Read the model definition and answer for the solid it produces. Units are mm, in the model's axes. Face numbers are marked on the shaded views. A direction names the side the tool comes from. Round coordinates to 2 decimals unless told otherwise and drop trailing zeros. Loops run counter-clockwise (first coordinate to the right, second up) from the corner with the lowest first, then second, coordinate; pieces in that order, holes last. Notation, with made-up numbers: M 46.25,-12.5 L 82.25,-12.5 A12 cw 82.25,-6.5 Z; hole C 38.25,-10.5 d7. An arc over 180 degrees is marked long. Write each question's results on one line, items separated by ' | '.
from build123d import *

# Parameters (mm, degrees)
SKETCH2_W           = 57
SKETCH2_H           = 120.75
SKETCH2_W_2         = 51
SKETCH2_H_2         = 114.75
BOSS_EXTRUDE1_DEPTH = 75
SKETCH3_W           = 57
SKETCH3_H           = 120.75
BOSS_EXTRUDE2_DEPTH = 3
SKETCH4_W           = 78
SKETCH4_H           = 57
BOSS_EXTRUDE3_DEPTH = 5
SKETCH6_R           = 2.675
CUT_EXTRUDE2_DEPTH  = 10
CUT_EXTRUDE3_DEPTH  = 138.287528874
BOSS_EXTRUDE4_REACH = 139.288
CUT_EXTRUDE7_DEPTH  = 150.745739841
BOSS_EXTRUDE8_DEPTH = 5
SKETCH21_R          = 3
CUT_EXTRUDE11_DEPTH = 1094
CHAMFER2_SIZE       = 2
CHAMFER2_SIZE2      = 6.751886845
SKETCH22_R          = 1.675
CUT_EXTRUDE12_DEPTH = 1094
CUT_EXTRUDE13_DEPTH = 5
SKETCH25_R          = 5.125
CUT_EXTRUDE14_DEPTH = 131.551099899
CHAMFER3_SIZE       = 2
FILLET1_R           = 2
SKETCH27_R          = 3
CUT_EXTRUDE15_DEPTH = 3
CUT_EXTRUDE16_DEPTH = 10


with BuildPart() as part:
    # Sketch2 → Boss-Extrude1 (new body)
    with BuildSketch(Plane(origin=(0, 0, 0), x_dir=(0, 0, -1), z_dir=(1, 0, 0))):
        with Locations((2.896243414, -39.494242434)):
            Rectangle(SKETCH2_W, SKETCH2_H)
        with Locations((2.896243414, -39.494242434)):
            Rectangle(SKETCH2_W_2, SKETCH2_H_2, mode=Mode.SUBTRACT)
    extrude(amount=BOSS_EXTRUDE1_DEPTH)

    # Sketch3 → Boss-Extrude2 (add)
    with BuildSketch(Plane.ZY):
        with Locations((-2.896243414, -39.494242434)):
            Rectangle(SKETCH3_W, SKETCH3_H)
    extrude(amount=BOSS_EXTRUDE2_DEPTH)

    # Sketch4 → Boss-Extrude3 (add)
    with BuildSketch(Plane(origin=(0, 20.880757566, 0), x_dir=(1, 0, 0), z_dir=(0, 1, 0))):
        with Locations((36, 2.896243414)):
            Rectangle(SKETCH4_W, SKETCH4_H)
    extrude(amount=BOSS_EXTRUDE3_DEPTH)

    # Sketch6 → Cut-Extrude2 (cut)
    with BuildSketch(Plane(origin=(0, 25.880757566, 0), x_dir=(1, 0, 0), z_dir=(0, 1, 0))):
        with Locations(Location((36, 18.896243414, 0), (0, 0, 270))):
            Circle(SKETCH6_R)
        with Locations(Location((36, -13.103756586, 0), (0, 0, 90))):
            Circle(SKETCH6_R)
    extrude(amount=-CUT_EXTRUDE2_DEPTH, mode=Mode.SUBTRACT)

    # Sketch8 → Cut-Extrude3 (cut, through all)
    with BuildSketch(Plane(origin=(0, 0, -31.396243414), x_dir=(-1, 0, 0), z_dir=(0, 0, -1))):
        Polygon((3, -99.869242434), (3, -79.869242434), (-17, -99.869242434), align=None)
    extrude(amount=-CUT_EXTRUDE3_DEPTH, mode=Mode.SUBTRACT)

    # Sketch9 → Boss-Extrude4 (add, up to next)
    with BuildSketch(Plane.XY.offset(25.603756586), mode=Mode.PRIVATE) as boss_extrude4_sk1:
        Polygon((-3, -79.869242434), (17, -99.869242434), (21.242640687, -99.869242434), (-3, -75.626601747), align=None)
    boss_extrude4_tool1 = extrude(boss_extrude4_sk1.sketch, amount=-BOSS_EXTRUDE4_REACH, mode=Mode.PRIVATE) - part.part
    add(boss_extrude4_tool1.solids().sort_by_distance((8.094564, -88.774678, 25.603757))[0])

    # Sketch15 → Cut-Extrude7 (cut, through all)
    with BuildSketch(Plane.XZ.offset(99.869242434)):
        with BuildLine():
            Line((62.625, 7.228756586), (62.625, 11.978756586))
            ThreePointArc((62.625, 11.978756586), (65, 14.353756586), (67.375, 11.978756586))
            Line((67.375, 11.978756586), (67.375, 7.228756586))
            ThreePointArc((67.375, 7.228756586), (65, 4.853756586), (62.625, 7.228756586))
        make_face()
        with BuildLine():
            Line((63.643986667, -17.72757696), (63.643986667, -12.97757696))
            ThreePointArc((63.643986667, -12.97757696), (66.018986667, -10.60257696), (68.393986667, -12.97757696))
            Line((68.393986667, -12.97757696), (68.393986667, -17.72757696))
            ThreePointArc((68.393986667, -17.72757696), (66.018986667, -20.10257696), (63.643986667, -17.72757696))
        make_face()
    extrude(amount=-CUT_EXTRUDE7_DEPTH, mode=Mode.SUBTRACT)

    # Sketch20 → Boss-Extrude8 (add)
    with BuildSketch(Plane(origin=(0, 0, 0), x_dir=(0, 0, -1), z_dir=(1, 0, 0))):
        with BuildLine():
            Line((-9.103756586, 5.880757566), (-9.103756586, 17.880757566))
            Line((-9.103756586, 17.880757566), (14.896243414, 17.880757566))
            Line((14.896243414, 17.880757566), (14.896243414, 5.880757566))
            ThreePointArc((14.896243414, 5.880757566), (2.896243414, -6.119242434), (-9.103756586, 5.880757566))
        make_face()
    extrude(amount=BOSS_EXTRUDE8_DEPTH)

    # Sketch21 → Cut-Extrude11 (cut)
    with BuildSketch(Plane(origin=(5, 0, 0), x_dir=(0, 0, -1), z_dir=(1, 0, 0))):
        with Locations((2.896243414, 5.937348)):
            Circle(SKETCH21_R)
    extrude(amount=-CUT_EXTRUDE11_DEPTH, mode=Mode.SUBTRACT)

    # Chamfer2
    chamfer2_edges = [part.edges().sort_by_distance(p)[0] for p in [
        (5, 5.937348, 0.103756586),
    ]]
    chamfer2_side = [part.faces().sort_by_distance(p)[0] for p in [
        (5, 11.880757566, 8.764345331),
    ]]
    chamfer(chamfer2_edges, length=CHAMFER2_SIZE, length2=CHAMFER2_SIZE2, reference=chamfer2_side[0])

    # Sketch22 → Cut-Extrude12 (cut)
    with BuildSketch(Plane(origin=(5, 0, 0), x_dir=(0, 0, -1), z_dir=(1, 0, 0))):
        with Locations((-5.603756586, 5.880757566)):
            Circle(SKETCH22_R)
        with Locations((11.396243414, 5.880757566)):
            Circle(SKETCH22_R)
    extrude(amount=-CUT_EXTRUDE12_DEPTH, mode=Mode.SUBTRACT)

    # Sketch24 → Cut-Extrude13 (cut)
    with BuildSketch(Plane.XZ.offset(-17.880757566)):
        Polygon((40.820874748, -18.896243414), (38.410437374, -14.721243414), (33.589562626, -14.721243414), (31.179125252, -18.896243414), (33.589562626, -23.071243414), (38.410437374, -23.071243414), align=None)
        Polygon((38.410437374, 17.278756586), (40.820874748, 13.103756586), (38.410437374, 8.928756586), (33.589562626, 8.928756586), (31.179125252, 13.103756586), (33.589562626, 17.278756586), align=None)
    extrude(amount=-CUT_EXTRUDE13_DEPTH, mode=Mode.SUBTRACT)

    # Sketch25 → Cut-Extrude14 (cut, through all)
    with BuildSketch(Plane.ZY.offset(3)):
        with Locations((-2.896243414, -26.994242434)):
            Circle(SKETCH25_R)
    extrude(amount=-CUT_EXTRUDE14_DEPTH, mode=Mode.SUBTRACT)

    # Chamfer3
    chamfer3_edges = [part.edges().sort_by_distance(p)[0] for p in [
        (-3, -26.994242434, -31.396243414),
        (-3, 25.880757566, -2.896243414),
        (-3, -26.994242434, 25.603756586),
    ]]
    chamfer(chamfer3_edges, length=CHAMFER3_SIZE)

    # Fillet1
    # the kernel refuses this fillet: 2 mm, written as the material it takes off along each edge
    with BuildSketch(Plane(origin=(-3, 5.937348, -2.896243414), x_dir=(0, 0, -1), z_dir=(0, -1, 0))) as fillet1_piece_1:
        with BuildLine():
            CenterArc((4.853285238, 2), FILLET1_R, 202.082634117, 67.917365883)
            Line((3, 1.248113155), (2.962934295, 1.233075418))
            ThreePointArc((2.962934295, 1.233075418), (2.96, 0.624056577), (2.96, 0))
            Line((2.96, 0), (3, -0.04))
            Line((3, -0.04), (4.853285238, -0.04))
            Line((4.853285238, -0.04), (4.853285238, 0))
        make_face()
    revolve(axis=Axis((-3, 5.937348, -2.896243414), (1, 0, 0)), mode=Mode.SUBTRACT)

    # Sketch27 → Cut-Extrude15 (cut)
    with BuildSketch(Plane.ZY.offset(3)):
        with Locations((-11.396243414, 5.880757566)):
            Circle(SKETCH27_R)
        with Locations((5.603756586, 5.880757566)):
            Circle(SKETCH27_R)
    extrude(amount=-CUT_EXTRUDE15_DEPTH, mode=Mode.SUBTRACT)

    # Sketch28 → Cut-Extrude16 (cut)
    with BuildSketch(Plane(origin=(0, 0, -31.396243414), x_dir=(-1, 0, 0), z_dir=(0, 0, -1))):
        with BuildLine():
            Line((-75, 9.880757566), (-75, -44.707153183))
            ThreePointArc((-75, -44.707153183), (-55.8, -17.413197809), (-75, 9.880757566))
        make_face()
    extrude(amount=-CUT_EXTRUDE16_DEPTH, mode=Mode.SUBTRACT)


solid = part.part
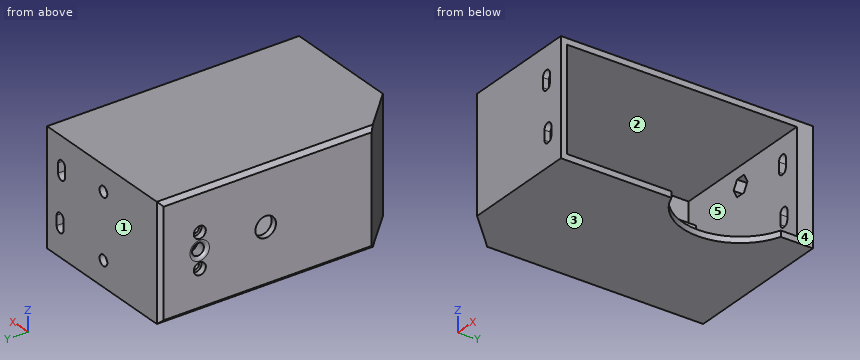
Item 1: The part is cut by section A-A (x = 36). Determine the outline of the cut face in (y, z), plus the area to 3 significant figures.
Outcome:
outline: M -99.87,-31.4 L 25.88,-31.4 L 25.88,-21.57 L 22.88,-21.57 L 22.88,-23.07 L 17.88,-23.07 L 17.88,-28.4 L -96.87,-28.4 L -96.87,22.6 L 17.88,22.6 L 17.88,17.28 L 22.88,17.28 L 22.88,15.78 L 25.88,15.78 L 25.88,25.6 L -99.87,25.6 Z; M 17.88,-14.72 L 22.88,-14.72 L 22.88,-16.22 L 25.88,-16.22 L 25.88,10.43 L 22.88,10.43 L 22.88,8.93 L 17.88,8.93 Z | area: 1,200 mm2
Item 2: Straight lines are drawn through the part: line 1 (Z direction, x = 59.5, y = -84); line 2 (Y direction, x = 60.5, z = -23.5); line 3 (X direction, y = -24, z = 7). For each, find the intervals that lie inside material, in ascending order.
Outcome:
line 1: z = -31.4 to -28.4, 22.6 to 25.6 | line 2: y = -99.87 to -96.87, 17.88 to 25.88 | line 3: x = -3 to 0
Item 3: Flat-ended cylindrical pins translate along their axes: pin 1 (12 mm diameter, centred on y = 8.5, z = -8.5, fed in from +X); pin 2 (1 mm diameter, centred on y = -32.5, z = -8, fed in from +X); pin 3 (3.5 mm diameter, centred on y = -98, z = -15.5, fed in from -X). Find the tip coordinate at first contact, or state that the pin passes through.
Outcome:
pin 1: stops at x = 5 | pin 2: stops at x = 0 | pin 3: stops at x = 13.38
Item 4: The mould has two halves that part along Y. Classify the marked faces 1, 2 and 3: pulls with the +Y half, pulls with the -Y half, needs draft (parallel to the pull), parting line crosses it, or undercut.
Outcome:
face 1: pulls with the +Y half | face 2: undercut | face 3: needs draft
Item 5: For the marked faces 4 and 5, determine the directions among +Z, -Z, +X, -X, +Y, -Y from which every point of the face is accessible in a straight line to the end or side of a thin tool.
Outcome:
face 4: +Z, -Z, +X, +Y, -Y | face 5: +X
Item 6: The part is cut by section D-D (x = 65). Determine the outline of the cut face in (y, z).
Outcome:
outline: M -99.87,-31.4 L -38.6,-31.4 L -38.6,-28.4 L -96.87,-28.4 L -96.87,-19.87 L -99.87,-19.87 Z; M -99.87,-10.83 L -96.87,-10.83 L -96.87,4.85 L -99.87,4.85 Z; M -99.87,14.35 L -96.87,14.35 L -96.87,22.6 L 17.88,22.6 L 17.88,14.35 L 25.88,14.35 L 25.88,25.6 L -99.87,25.6 Z; M 3.78,-31.4 L 25.88,-31.4 L 25.88,-19.87 L 17.88,-19.87 L 17.88,-28.4 L 3.78,-28.4 Z; M 17.88,-10.83 L 25.88,-10.83 L 25.88,4.85 L 17.88,4.85 Z
Item 7: The part is cut by section C-C (y = -77). Determine the outline of the cut face in (x, z), plus the area to 3 significant figures.
Outcome:
outline: M -3,-29.4 L -1,-31.4 L 75,-31.4 L 75,-28.4 L 0,-28.4 L 0,22.6 L 75,22.6 L 75,25.6 L -1,25.6 L -3,23.6 Z | area: 617 mm2
Item 8: The part is cut by section B-B (x = 28). Determine the outline of the cut face in (y, z).
Outcome:
outline: M -99.87,-31.4 L 25.88,-31.4 L 25.88,25.6 L -99.87,25.6 Z; hole M -96.87,-28.4 L 17.88,-28.4 L 17.88,22.6 L -96.87,22.6 Z
